```python
from build123d import *

# Parameters (mm, degrees)
EXTRUDE1_DEPTH = 4.6
SKETCH2_R      = 1
EXTRUDE2_DEPTH = 1
SKETCH3_R      = 1
EXTRUDE3_DEPTH = 1


with BuildPart() as part:
    # Sketch1 → Extrude1 (new body)
    with BuildSketch(Plane(origin=(0, 0, 0), x_dir=(0, 0, -1), z_dir=(1, 0, 0))):
        with BuildLine():
            Line((28.351631804, 12.38738065), (28.351631804, 5.88738065))
            Line((28.351631804, 5.88738065), (27.351631804, 4.88738065))
            Line((27.351631804, 4.88738065), (19.851631804, 4.88738065))
            Line((19.851631804, 4.88738065), (18.851631804, 5.88738065))
            Line((18.851631804, 5.88738065), (18.851631804, 12.38738065))
            Line((18.851631804, 12.38738065), (12.476631804, 12.38738065))
            Line((12.476631804, 12.38738065), (12.476631804, 43.38738065))
            Line((12.476631804, 43.38738065), (5.976631804, 43.38738065))
            Line((5.976631804, 43.38738065), (4.976631804, 44.38738065))
            Line((4.976631804, 44.38738065), (4.976631804, 62.38738065))
            Line((4.976631804, 62.38738065), (5.976631804, 63.38738065))
            Line((5.976631804, 63.38738065), (12.476631804, 63.38738065))
            Line((12.476631804, 63.38738065), (12.476631804, 80.13738065))
            Line((12.476631804, 80.13738065), (16.976631804, 80.13738065))
            Line((16.976631804, 80.13738065), (16.976631804, 79.13738065))
            Line((16.976631804, 79.13738065), (19.476631804, 79.13738065))
            Line((19.476631804, 79.13738065), (19.476631804, 80.13738065))
            Line((19.476631804, 80.13738065), (24.476631804, 80.13738065))
            Line((24.476631804, 80.13738065), (24.476631804, 83.63738065))
            Line((24.476631804, 83.63738065), (19.476631804, 83.63738065))
            Line((19.476631804, 83.63738065), (19.476631804, 84.63738065))
            Line((19.476631804, 84.63738065), (16.976631804, 84.63738065))
            Line((16.976631804, 84.63738065), (16.976631804, 83.63738065))
            Line((16.976631804, 83.63738065), (12.476631804, 83.63738065))
            Line((12.476631804, 83.63738065), (12.476631804, 88.38738065))
            ThreePointArc((12.476631804, 88.38738065), (14.233991117, 92.630021337), (18.476631804, 94.38738065))
            Line((18.476631804, 94.38738065), (49.976631804, 94.38738065))
            ThreePointArc((49.976631804, 94.38738065), (54.219272491, 92.630021337), (55.976631804, 88.38738065))
            Line((55.976631804, 88.38738065), (55.976631804, 69.38738065))
            Line((55.976631804, 69.38738065), (52.476631804, 66.38738065))
            Line((52.476631804, 66.38738065), (52.476631804, 12.38738065))
            Line((52.476631804, 12.38738065), (46.101631804, 12.38738065))
            Line((46.101631804, 12.38738065), (46.101631804, 5.88738065))
            Line((46.101631804, 5.88738065), (45.101631804, 4.88738065))
            Line((45.101631804, 4.88738065), (37.601631804, 4.88738065))
            Line((37.601631804, 4.88738065), (36.601631804, 5.88738065))
            Line((36.601631804, 5.88738065), (36.601631804, 12.38738065))
            Line((36.601631804, 12.38738065), (34.226631804, 12.38738065))
            Line((34.226631804, 12.38738065), (34.226631804, 16.88738065))
            Line((34.226631804, 16.88738065), (35.226631804, 16.88738065))
            Line((35.226631804, 16.88738065), (35.226631804, 19.38738065))
            Line((35.226631804, 19.38738065), (34.226631804, 19.38738065))
            Line((34.226631804, 19.38738065), (34.226631804, 24.38738065))
            Line((34.226631804, 24.38738065), (30.726631804, 24.38738065))
            Line((30.726631804, 24.38738065), (30.726631804, 19.38738065))
            Line((30.726631804, 19.38738065), (29.726631804, 19.38738065))
            Line((29.726631804, 19.38738065), (29.726631804, 16.88738065))
            Line((29.726631804, 16.88738065), (30.726631804, 16.88738065))
            Line((30.726631804, 16.88738065), (30.726631804, 12.38738065))
            Line((30.726631804, 12.38738065), (28.351631804, 12.38738065))
        make_face()
    extrude(amount=EXTRUDE1_DEPTH)

    # Sketch2 → Extrude2 (cut)
    with BuildSketch(Plane.XY.offset(-24.476631804)):
        with Locations((2.3, 81.88738065)):
            Circle(SKETCH2_R)
    extrude(amount=-EXTRUDE2_DEPTH, mode=Mode.SUBTRACT)

    # Sketch3 → Extrude3 (cut)
    with BuildSketch(Plane.XZ.offset(-24.38738065)):
        with Locations(Location((2.3, -32.476631804, 0), (0, 0, 270))):
            Circle(SKETCH3_R)
    extrude(amount=-EXTRUDE3_DEPTH, mode=Mode.SUBTRACT)


solid = part.part
```
Geometry: final body of the model. Coordinates: model frame, mm. A direction names the side the tool comes from. Coordinates: 2 decimals unless noted, no trailing zeros. Order: outer loops, then holes, each group sorted by start corner. A loop starts at its lowest first (then second) coordinate and runs counter-clockwise, first axis right, second up. Notation, with made-up numbers: (-29.75, -20) -> (15.25, -20) arc R20 ccw to (15.25, 19) -> close; hole circle Ø1 at (86.25, 39.25). An arc over 180 degrees is marked (long way). Use CSV: the item, a comma, the result in double quotes.
1) Pin query (flat end, axial travel): pin 1 Ø1.1 at (x, y) = (3, 84) entering from +Z; pin 2 Ø2.5 at (x, y) = (1.5, 9) entering from -Z; pin 3 Ø0.8 at (x, z) = (2, -17.5) entering from +Y. Return the tip coordinate at first contact, or that it passes through.
Findings:
pin 1,"stops at z = -12.48"
pin 2,"stops at z = -46.1"
pin 3,"stops at y = 94.36"
2) Section A-A on y = 14. Output: boundary loops of the cut face in (x, z).
Findings:
outline,"(0, -52.48) -> (4.6, -52.48) -> (4.6, -34.23) -> (0, -34.23) -> close; (0, -30.73) -> (4.6, -30.73) -> (4.6, -12.48) -> (0, -12.48) -> close"
3) Section C-C on y = 86.5. Output: boundary loops of the cut face in (x, z), then the cut area to 3 significant figures.
Findings:
outline,"(0, -55.98) -> (4.6, -55.98) -> (4.6, -12.48) -> (0, -12.48) -> close"
area,"200 mm^2"
4) Mould query, pull axis Z, two halves, no side actions, for faces 4 (the flat face through (2, 18, -29.727)), 5 (the flat face through (2, 9, -28.352)), 6 (the cylindrical face through (2.27, 92.68, -54.17)), 7 (the flat face through (2, 80.137, -22)). Classes: +Z half, -Z half, draft (parallel to the pull), parting line (faces both ways), or undercut.
Findings:
face 4,"undercut"
face 5,"undercut"
face 6,"-Z half"
face 7,"draft"
5) Line query: line 1 (Y direction, x = 2.3, z = -24.85); line 2 (Z direction, x = 2.2, y = 22.5); line 3 (Y direction, x = 3.4, z = -22). Output: solid intervals per line, ascending.
Findings:
line 1,"y = 4.89 to 80.89, 82.89 to 94.39"
line 2,"z = -52.48 to -34.23, -30.73 to -12.48"
line 3,"y = 4.89 to 80.14, 83.64 to 94.39"
6) Section B-B on y = 58. Output: boundary loops of the cut face in (x, z), then the cut area to 4 significant figures.
Findings:
outline,"(0, -52.48) -> (4.6, -52.48) -> (4.6, -4.98) -> (0, -4.98) -> close"
area,"218.5 mm^2"
7) Access query for faces 1 (the flat face through (1, 82, -24.477)), 2 (the cylindrical face through (2.17, 82.88, -24.97)), 3 (the flat face through (1, 24.387, -33)). Directions: +Z, -Z, +X, -X, +Y, -Y. A direction counts if a zero-diameter tool reaches every point of the face in a straight line with its end or side. Return the directions, or none.
Findings:
face 1,"+Z, +X, -X"
face 2,"+Z"
face 3,"+X, -X, -Y"
